CAD build for the part. Positions are in the model's coordinates, mm. Face numbers are marked on the shaded views. Coordinates: 2 decimals unless noted, no trailing zeros. Loops run counter-clockwise (first coordinate to the right, second up) from the corner with the lowest first, then second, coordinate; pieces in that order, holes last. Notation, with made-up numbers: (-34, 54.25) - (19, 54.25) arc R18 ccw to (19, 89.25) - close; hole circle Ø2 at (-10, 47). An arc over 180 degrees is marked (long way). Put each result on its own line as item: value.
```python
from build123d import *

# Parameters (mm, degrees)
F0_W     = 60
F0_H     = 80
F1_DEPTH = 12
F2_R     = 10
F3_DEPTH = 25
F4_SIZE  = 1.5


with BuildPart() as f1:
    # F0 (on Top) → F1 (new body)
    with BuildSketch(Plane.XY):
        with Locations((-1.378186, -7.605234)):
            Rectangle(F0_W, F0_H)
    extrude(amount=F1_DEPTH)

    # F2 (on face) → F3 (cut)
    with BuildSketch(Plane.XY.offset(12)):
        with Locations((-13.878186, 0)):
            Circle(F2_R)
    extrude(amount=-F3_DEPTH, mode=Mode.SUBTRACT)

    # F4
    f4_edges = [f1.edges().sort_by_distance(p)[0] for p in [
        (-23.878186, 0, 12),
        (-31.378186, -7.605234, 12),
        (-1.378186, 32.394766, 12),
        (-1.378186, 32.394766, 0),
        (28.621814, -7.605234, 0),
        (-31.378186, -7.605234, 0),
        (-1.378186, -47.605234, 0),
        (-23.878186, 0, 0),
        (28.621814, -7.605234, 12),
        (-1.378186, -47.605234, 12),
        (28.621814, -47.605234, 6),
        (28.621814, 32.394766, 6),
        (-31.378186, -47.605234, 6),
    ]]
    chamfer(f4_edges, length=F4_SIZE)


solid = f1.part
```
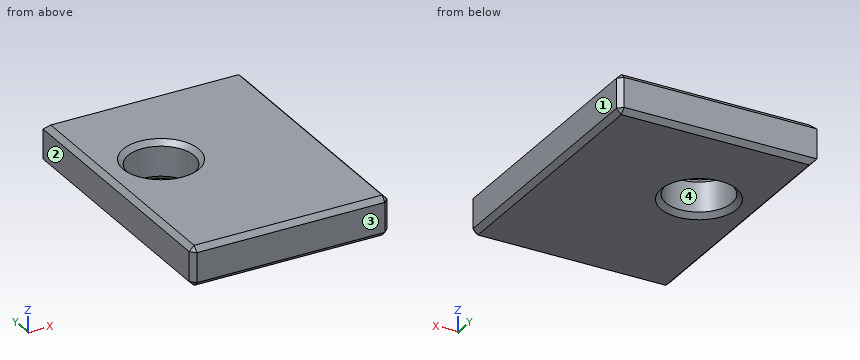
Q1. Slice it at B-B, the plane z = 9. Give the cut face in (x, y), then the cut area to 3 significant figures.
Determined:
outline: (-31.38, -46.11) - (-29.88, -47.61) - (27.12, -47.61) - (28.62, -46.11) - (28.62, 30.89) - (27.12, 32.39) - (-31.38, 32.39) - close; hole circle Ø20 at (-13.88, 0)
area: 4,480 mm2
Q2. Wall check: L1, parallel to Y at x = -14.5, z = 4.25; L2, parallel to Y at x = -18, z = 7; L3, parallel to X at y = -5.5, z = 10.5. Give the ranges that are in metal, low to high. Write a range as from..to.
Determined:
L1: -47.61..-9.98, 9.98..32.39
L2: -47.61..-9.11, 9.11..32.39
L3: -31.38..-22.23, -5.53..28.62
Q3. Slice it at A-A, the plane y = 0. Give the cut face in (x, z).
Determined:
outline: (-31.38, 1.5) - (-29.88, 0) - (-25.38, 0) - (-23.88, 1.5) - (-23.88, 10.5) - (-25.38, 12) - (-29.88, 12) - (-31.38, 10.5) - close; (-3.88, 1.5) - (-2.38, 0) - (27.12, 0) - (28.62, 1.5) - (28.62, 10.5) - (27.12, 12) - (-2.38, 12) - (-3.88, 10.5) - close
Q4. Mould opens along X. For the marked faces 1, 2, 3 and 4 say: +X half, -X half, draft (parallel to the pull), parting line (faces both ways), or undercut.
Determined:
face 1: +X half
face 2: -X half
face 3: draft
face 4: undercut
